The figure shows three views and two pictorial views of one solid part (mm, origin at its lowest corner). Answer the questions. Round coordinates to 2 decimals unless told otherwise and drop trailing zeros. Loops run counter-clockwise (first coordinate to the right, second up) from the corner with the lowest first, then second, coordinate; pieces in that order, holes last. Notation, with made-up numbers: (-36, 85) -> (7, 85) arc R28 ccw to (7, 124) -> close; hole circle Ø7 at (63.5, 23). An arc over 180 degrees is marked (long way). Write each question's results on one line, items separated by ' | '. Start each with the question number.
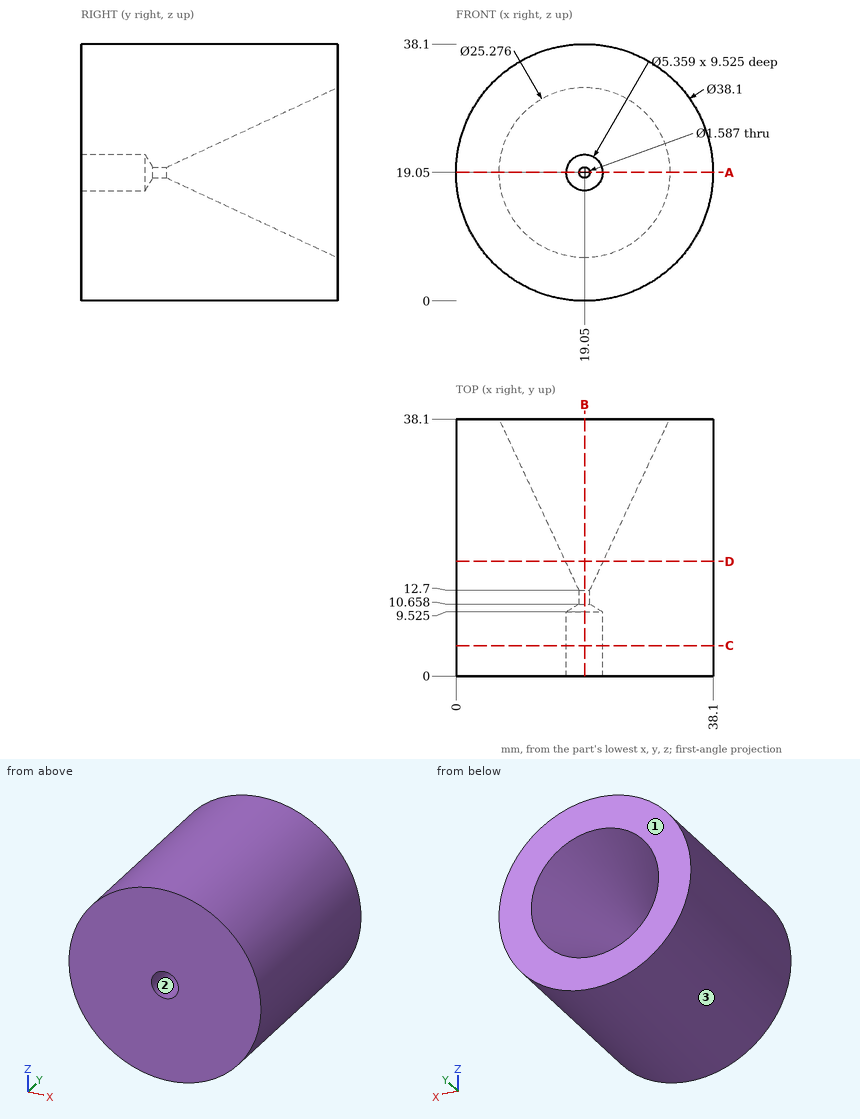
Item 1: Straight lines are drawn through the part: L1, parallel to X at y = 11, z = 19; L2, parallel to Z at x = 19, y = 6. For each, find the intervals that lie inside material, in ascending order. Write a range as [from, to].
Item 2: The part is cut by section A-A, the plane z = 19.05. Give the vertices of the cut face in (x, y) (1 decimal), plus the area to 3 significant figures.
Item 3: The part is cut by section C-C, the plane y = 4.5. Give the vertices of the cut face in (x, z), plus the area to 3 significant figures.
Item 4: The part is cut by section D-D, the plane y = 17. Give the vertices of the cut face in (x, z), plus the area to 3 significant figures.
Item 5: Each of these flat-tipped pins is pushed along its axis until it touches: pin 1 Ø2 at (x, y) = (4, 18.5) entering from -Z (1 decimal); pin 2 Ø2 at (y, z) = (26, 19) entering from +X; pin 3 Ø4 at (y, z) = (18.5, 5.5) entering from -X. Where does it stop, or does it pass through?
Item 6: The part is cut by section B-B, the plane x = 19.05. Give the vertices of the cut face in (y, z) (1 decimal).
Item 7: Determine the mould class of the marked faces 1, 2 and 3 for opening direction X: +X half, -X half, draft (parallel to the pull), parting line (faces both ways), or undercut.
Report:
1) L1: x = [0, 18.26], [19.84, 38.1] | L2: z = [0, 16.37], [21.73, 38.1]
2) outline: (0, 0) -> (16.4, 0) -> (16.4, 9.5) -> (18.3, 10.7) -> (18.3, 12.7) -> (6.4, 38.1) -> (0, 38.1) -> close; (19.8, 10.7) -> (21.7, 9.5) -> (21.7, 0) -> (38.1, 0) -> (38.1, 38.1) -> (31.7, 38.1) -> (19.8, 12.7) -> close | area: 1,050 mm2
3) outline: circle Ø38.1 at (19.05, 19.05); hole circle Ø5.36 at (19.05, 19.05) | area: 1,120 mm2
4) outline: circle Ø38.1 at (19.05, 19.05); hole circle Ø5.6 at (19.05, 19.05) | area: 1,120 mm2
5) pin 1: stops at z = 6.2 | pin 2: stops at x = 38.1 | pin 3: stops at x = 3.9
6) outline: (0, 0) -> (38.1, 0) -> (38.1, 6.4) -> (12.7, 18.3) -> (10.7, 18.3) -> (9.5, 16.4) -> (0, 16.4) -> close; (0, 21.7) -> (9.5, 21.7) -> (10.7, 19.8) -> (12.7, 19.8) -> (38.1, 31.7) -> (38.1, 38.1) -> (0, 38.1) -> close
7) face 1: draft | face 2: undercut | face 3: parting line
